```python
from build123d import *

# Parameters (mm, degrees)
SKETCH_1_W          = 90.6
SKETCH_1_H          = 50
SKETCH_1_W_2        = 80.6
SKETCH_1_H_2        = 40
EXTRUDE_1_DEPTH     = 6
FILLET_1_R          = 1
SKETCH_2_R          = 2
CUT_EXTRUDE_1_DEPTH = 95.177279638
SKETCH_3_R          = 1.5
CUT_EXTRUDE_2_DEPTH = 68.73544124


with BuildPart() as part:
    # 草图1 → 凸台-拉伸1 (new body)
    with BuildSketch(Plane.XY):
        Rectangle(SKETCH_1_W, SKETCH_1_H)
        Rectangle(SKETCH_1_W_2, SKETCH_1_H_2, mode=Mode.SUBTRACT)
    extrude(amount=EXTRUDE_1_DEPTH)

    # 圆角1
    fillet_1_edges = [part.edges().sort_by_distance(p)[0] for p in [
        (40.3, -20, 3),
        (40.3, 20, 3),
        (-40.3, 20, 3),
        (-40.3, -20, 3),
    ]]
    fillet(fillet_1_edges, radius=FILLET_1_R)

    # 草图2 → 切除-拉伸1 (cut, through all)
    with BuildSketch(Plane(origin=(45.3, 0, 0), x_dir=(0, 0, -1), z_dir=(1, 0, 0))):
        with Locations((-3, 15)):
            Circle(SKETCH_2_R)
        with Locations((-3, -15)):
            Circle(SKETCH_2_R)
    extrude(amount=-CUT_EXTRUDE_1_DEPTH, mode=Mode.SUBTRACT)

    # 草图3 → 切除-拉伸2 (cut, through all)
    with BuildSketch(Plane(origin=(0, 25, 0), x_dir=(1, 0, 0), z_dir=(0, 1, 0))):
        with Locations(Location((-25.3, -3, 0), (0, 0, 270))):
            Circle(SKETCH_3_R)
        with Locations(Location((25.3, -3, 0), (0, 0, 270))):
            Circle(SKETCH_3_R)
    extrude(amount=-CUT_EXTRUDE_2_DEPTH, mode=Mode.SUBTRACT)


solid = part.part
```
For this review, take the finished solid that the model builds, in its own axes (mm). A direction names the side the tool comes from. Give positions to 0.01 mm unless a question says otherwise; leave off trailing zeros. Write each loop counter-clockwise with the first axis right and the second up, starting at its lowest first coordinate (ties: lowest second). Pieces come first, ordered by that corner, then holes. Notation, with made-up numbers: M 23.5,64.25 L 30.5,64.25 A28 ccw 30.5,100.25 Z; hole C -4.75,77 d10. An arc over 180 degrees is marked long. One line per item, written item: value.
1) The part is to be moulded in two halves that separate along Y. For faces 3 (the flat face through (-1, -25, 3)), 4 (the flat face through (-1, 25, 3)), 5 (the cylindrical face through (-43, 17, 3)), 6 (the flat face through (45.3, 0, 3)), say which applies: +Y half, -Y half, draft (parallel to the pull), parting line (faces both ways), or undercut.
Results are:
face 3: -Y half
face 4: +Y half
face 5: undercut
face 6: draft
2) Take a section at D-D, the plane x = -36. Write out the cut boundary in (y, z).
Results are:
outline: M -25,0 L -20,0 L -20,6 L -25,6 Z; M 20,0 L 25,0 L 25,6 L 20,6 Z
3) Take a section at B-B, the plane y = 12. Write out the cut boundary in (x, z).
Results are:
outline: M -45.3,0 L -40.3,0 L -40.3,6 L -45.3,6 Z; M 40.3,0 L 45.3,0 L 45.3,6 L 40.3,6 Z
4) For P1, Ø3.5, axis at y = -15, z = 3, coming from the -X side, flat-tipped, find the tip position at first contact; note if it passes through.
Results are:
P1: passes through
5) Take a section at C-C, the plane x = 25.3. Write out the cut boundary in (y, z).
Results are:
outline: M -25,0 L -20,0 L -20,1.5 L -25,1.5 Z; M -25,4.5 L -20,4.5 L -20,6 L -25,6 Z; M 20,0 L 25,0 L 25,1.5 L 20,1.5 Z; M 20,4.5 L 25,4.5 L 25,6 L 20,6 Z
6) For line 1 (X direction, y = 21.2, z = 3); line 2 (Y direction, x = -39, z = 4.7); line 3 (X direction, y = 15, z = 0.5), list the stretches that pass through material, from the lowest coordinate up. Write a range as from..to.
Results are:
line 1: x = -45.3..-26.8, -23.8..23.8, 26.8..45.3
line 2: y = -25..-20, 20..25
line 3: x = -45.3..-40.3, 40.3..45.3
7) For faces 1 (the cylindrical face through (43, 17, 3)), 2 (the flat face through (-40.3, 0, 3)), list the 3-axis set-ups (+Z, -Z, +X, -X, +Y, -Y) from which the entire face can be reached by the end or side of a thin tool; tool diameter is ignored.
Results are:
face 1: +X, -X
face 2: +Z, -Z
8) Take a section at A-A, the plane y = -15. Write out the cut boundary in (x, z).
Results are:
outline: M -45.3,0 L -40.3,0 L -40.3,1 L -45.3,1 Z; M -45.3,5 L -40.3,5 L -40.3,6 L -45.3,6 Z; M 40.3,0 L 45.3,0 L 45.3,1 L 40.3,1 Z; M 40.3,5 L 45.3,5 L 45.3,6 L 40.3,6 Z
